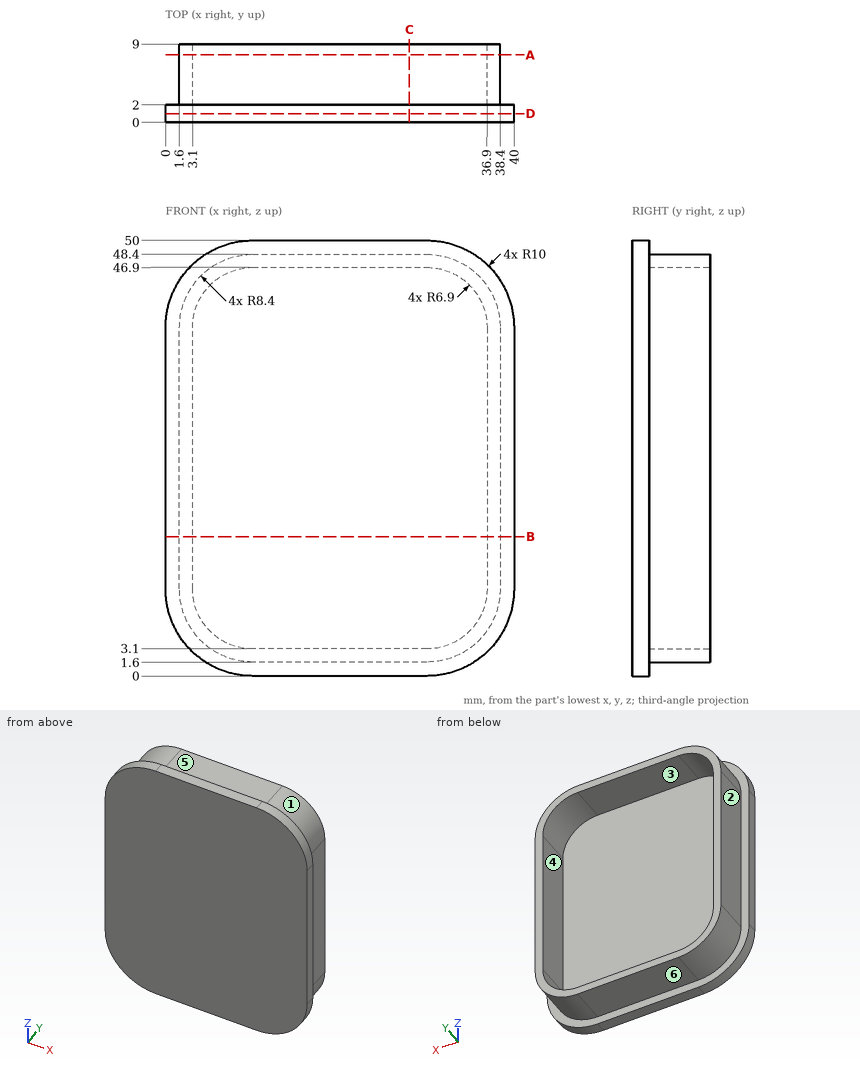
Can you work these out from the drawing? Everything is in mm from the part's minimum corner. A direction names the side the tool comes from. Round coordinates to 2 decimals unless told otherwise and drop trailing zeros. Loops run counter-clockwise (first coordinate to the right, second up) from the corner with the lowest first, then second, coordinate; pieces in that order, holes last. Notation, with made-up numbers: (31, -1) - (48, -1) arc R19 cw to (48, 34) - close; hole circle Ø7 at (67.25, 57.25). An arc over 180 degrees is marked (long way). Answer in a Markdown table with one row per item. Add a question column.
Q1. I want a section at B-B on z = 16. List the corners of the cut face in (x, y) for me.
Q2. I want a section at A-A on y = 7.75. List the corners of the cut face in (x, z) for me.
Q3. I want a section at D-D on y = 1. List the corners of the cut face in (x, z) for me, and give its area (3 significant figures).
Q4. We'd pull the mould along Z, two halves only. Please class the marked faces 1, 2 and 3: pulls with the +Z half, pulls with the -Z half, needs draft (parallel to the pull), parting line crosses it, or undercut.
Q5. I need wall thicknesses on L1, parallel to Z at x = 30, y = 7; L2, parallel to X at y = 5, z = 27.5; L3, parallel to Y at x = 22, z = 35. Which ranges of each line are inside material? Lowest first, please.
Q6. I want a section at C-C on x = 28. List the corners of the cut face in (y, z) for me.
Q7. Which directions (+Z, -Z, +X, -X, +Y, -Y) give clear straight access to the entire face, cutting with the end or side of a thin tool? Please do the marked faces 4, 5 and 6.
Q8. For pin 1 Ø2 at (x, z) = (25, 36) entering from +Y; pin 2 Ø2 at (y, z) = (5, 29.5) entering from +X; pin 3 Ø3.5 at (y, z) = (6, 31.5) entering from -X, each with a flat end and sliding along its axis, tell me the tip position at first contact or that it passes through.
A:
| question | item | result |
|---|---|---|
| 1 | outline | (0, 0) - (40, 0) - (40, 2) - (38.4, 2) - (38.4, 9) - (36.9, 9) - (36.9, 2) - (3.1, 2) - (3.1, 9) - (1.6, 9) - (1.6, 2) - (0, 2) - close |
| 2 | outline | (1.6, 10) arc R8.4 ccw to (10, 1.6) - (30, 1.6) arc R8.4 ccw to (38.4, 10) - (38.4, 40) arc R8.4 ccw to (30, 48.4) - (10, 48.4) arc R8.4 ccw to (1.6, 40) - close; hole (3.1, 10) arc R6.9 ccw to (10, 3.1) - (30, 3.1) arc R6.9 ccw to (36.9, 10) - (36.9, 40) arc R6.9 ccw to (30, 46.9) - (10, 46.9) arc R6.9 ccw to (3.1, 40) - close |
| 3 | outline | (0, 10) arc R10 ccw to (10, 0) - (30, 0) arc R10 ccw to (40, 10) - (40, 40) arc R10 ccw to (30, 50) - (10, 50) arc R10 ccw to (0, 40) - close |
| 3 | area | 1,910 mm^2 |
| 4 | face 1 | pulls with the +Z half |
| 4 | face 2 | needs draft |
| 4 | face 3 | undercut |
| 5 | L1 | 1.6 to 3.1, 46.9 to 48.4 |
| 5 | L2 | 1.6 to 3.1, 36.9 to 38.4 |
| 5 | L3 | 0 to 2 |
| 6 | outline | (0, 0) - (2, 0) - (2, 1.6) - (9, 1.6) - (9, 3.1) - (2, 3.1) - (2, 46.9) - (9, 46.9) - (9, 48.4) - (2, 48.4) - (2, 50) - (0, 50) - close |
| 7 | face 4 | +Y |
| 7 | face 5 | +Z, +X, -X, +Y |
| 7 | face 6 | -Z, +X, -X, +Y |
| 8 | pin 1 | y = 2 |
| 8 | pin 2 | x = 38.4 |
| 8 | pin 3 | x = 1.6 |
